Source: three-view drawing plus pictorial views. Frame: mm from the lowest corner of the part. A direction names the side the tool comes from. Give positions to 0.01 mm unless a question says otherwise; leave off trailing zeros. Order: outer loops, then holes, each group sorted by start corner. A loop starts at its lowest first (then second) coordinate and runs counter-clockwise, first axis right, second up.
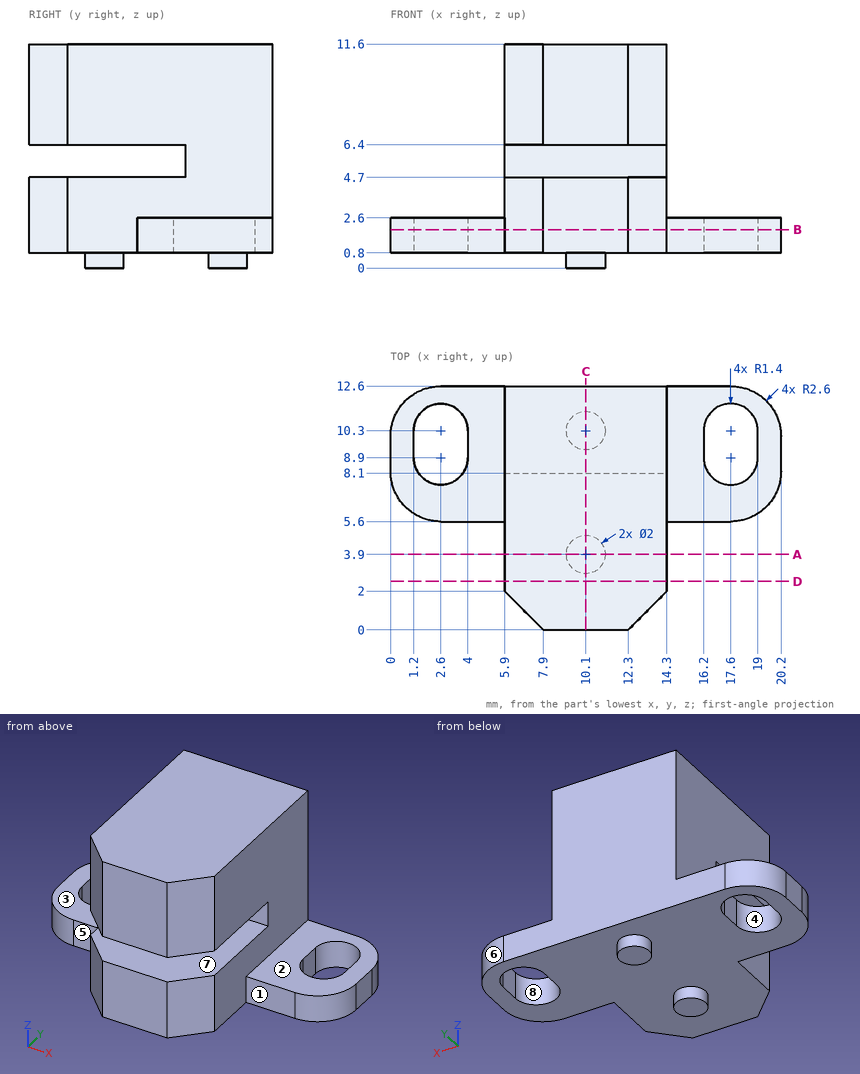
1) First-contact query: pin 1 Ø5.5 at (y, z) = (9.5, 7) entering from -X; pin 2 Ø3 at (y, z) = (7, 6) entering from +X; pin 3 Ø0.9 at (x, z) = (16, 2) entering from -Y. Flat tips, straight axial feed; report the tip coordinate or a pass-through.
Checks:
pin 1: stops at x = 5.9
pin 2: stops at x = 14.3
pin 3: stops at y = 5.6
2) Pull-direction query (X, two-part tool) for the marked faces 6, 7 and 8; classes: +X half, -X half, draft (parallel to the pull), parting line (faces both ways), or undercut.
Checks:
face 6: +X half
face 7: draft
face 8: undercut
3) Ray query, L1, parallel to Z at x = 11, y = 3; L2, parallel to X at y = 5.25, z = 7.25; L3, parallel to Y at x = 6, z = 5.75. Return the intervals inside material, ascending.
Checks:
L1: z = 0.8 to 4.7, 6.4 to 11.6
L2: x = 5.9 to 14.3
L3: y = 8.1 to 12.6
4) Section query C-C on x = 10.1. Output: boundary loops of the cut face in (y, z), and give its area (3 significant figures).
Checks:
outline: (0, 0.8) - (2.9, 0.8) - (2.9, 0) - (4.9, 0) - (4.9, 0.8) - (9.3, 0.8) - (9.3, 0) - (11.3, 0) - (11.3, 0.8) - (12.6, 0.8) - (12.6, 11.6) - (0, 11.6) - (0, 6.4) - (8.1, 6.4) - (8.1, 4.7) - (0, 4.7) - close
area: 126 mm2
5) Section query B-B on z = 2. Output: boundary loops of the cut face in (x, y), and give its area (3 significant figures).
Checks:
outline: (0, 8.2) arc R2.6 ccw to (2.6, 5.6) - (5.9, 5.6) - (5.9, 2) - (7.9, 0) - (12.3, 0) - (14.3, 2) - (14.3, 5.6) - (17.6, 5.6) arc R2.6 ccw to (20.2, 8.2) - (20.2, 10) arc R2.6 ccw to (17.6, 12.6) - (2.6, 12.6) arc R2.6 ccw to (0, 10) - close; hole (1.2, 8.9) arc R1.4 ccw to (4, 8.9) - (4, 10.3) arc R1.4 ccw to (1.2, 10.3) - close; hole (16.2, 8.9) arc R1.4 ccw to (19, 8.9) - (19, 10.3) arc R1.4 ccw to (16.2, 10.3) - close
area: 158 mm2
6) Section query A-A on y = 3.9. Output: boundary loops of the cut face in (x, z).
Checks:
outline: (5.9, 0.8) - (9.1, 0.8) - (9.1, 0) - (11.1, 0) - (11.1, 0.8) - (14.3, 0.8) - (14.3, 4.7) - (5.9, 4.7) - close; (5.9, 6.4) - (14.3, 6.4) - (14.3, 11.6) - (5.9, 11.6) - close
7) Reachability of the marked faces 1, 2, 3, 4 and 5 from +Z, -Z, +X, -X, +Y, -Y: full face, straight path, thin tool, end or side. Return the list, or none.
Checks:
face 1: +Z, -Z, +X, -Y
face 2: +Z, +X, +Y, -Y
face 3: +Z, -X, +Y, -Y
face 4: +Z, -Z
face 5: +Z, -Z, -X, -Y
8) Section query D-D on y = 2.5. Output: boundary loops of the cut face in (x, z).
Checks:
outline: (5.9, 0.8) - (14.3, 0.8) - (14.3, 4.7) - (5.9, 4.7) - close; (5.9, 6.4) - (14.3, 6.4) - (14.3, 11.6) - (5.9, 11.6) - close
